Design review of the part built by this model. Coordinates are the model's own, in mm. Face numbers are marked on the shaded views. A direction names the side the tool comes from. Give positions to 0.01 mm unless a question says otherwise; leave off trailing zeros. Order: outer loops, then holes, each group sorted by start corner. A loop starts at its lowest first (then second) coordinate and runs counter-clockwise, first axis right, second up. Notation, with made-up numbers: (64, 38) -> (116, 38) arc R9 ccw to (116, 47) -> close; hole circle Ø11 at (73.5, -27.75). An arc over 180 degrees is marked (long way). Use a Markdown table: item, result. Add a question column.
```python
from build123d import *

# Parameters (mm, degrees)
SKETCH1_W           = 20
SKETCH1_H           = 15
BOSS_EXTRUDE1_DEPTH = 2.54
SKETCH2_W           = 20
SKETCH2_H           = 2.54
BOSS_EXTRUDE2_DEPTH = 10.16
CUT_EXTRUDE1_REACH  = 20.933
SKETCH3_R           = 2.4765
FILLET1_R           = 2.54
SKETCH4_R           = 0.5
CUT_EXTRUDE2_DEPTH  = 10


with BuildPart() as part:
    # Sketch1 → Boss-Extrude1 (new body)
    with BuildSketch(Plane.XY):
        with Locations((0, 7.5)):
            Rectangle(SKETCH1_W, SKETCH1_H)
    extrude(amount=BOSS_EXTRUDE1_DEPTH)

    # Sketch2 → Boss-Extrude2 (add)
    with BuildSketch(Plane(origin=(0, 0, 0), x_dir=(-1, 0, 0), z_dir=(0, 0, -1))):
        with Locations((0, 1.27)):
            Rectangle(SKETCH2_W, SKETCH2_H)
    extrude(amount=BOSS_EXTRUDE2_DEPTH)

    # Sketch3 → Cut-Extrude1 (cut, up to next)
    with BuildSketch(Plane(origin=(0, 2.54, 0), x_dir=(1, 0, 0), z_dir=(0, 1, 0)), mode=Mode.PRIVATE) as cut_extrude1_sk1:
        with Locations(Location((0, 5.08, 0), (0, 0, 180))):
            Circle(SKETCH3_R)
    cut_extrude1_tool1 = extrude(cut_extrude1_sk1.sketch, amount=-CUT_EXTRUDE1_REACH, mode=Mode.PRIVATE) & part.part
    add(cut_extrude1_tool1.solids().sort_by_distance((0, 2.54, -5.08))[0], mode=Mode.SUBTRACT)

    # Fillet1
    fillet1_edges = [part.edges().sort_by_distance(p)[0] for p in [
        (0, 2.54, 0),
    ]]
    fillet(fillet1_edges, radius=FILLET1_R)

    # Sketch4 → Cut-Extrude2 (cut)
    with BuildSketch(Plane(origin=(0, 2.54, 0), x_dir=(1, 0, 0), z_dir=(0, 1, 0))):
        with Locations(Location((-8.35, 5.08, 0), (0, 0, 180))):
            Circle(SKETCH4_R)
        with Locations(Location((-4.35, 5.08, 0), (0, 0, 180))):
            Circle(SKETCH4_R)
        with Locations(Location((4.95, 5.08, 0), (0, 0, 180))):
            Circle(SKETCH4_R)
        with Locations(Location((8.95, 5.08, 0), (0, 0, 180))):
            Circle(SKETCH4_R)
    extrude(amount=-CUT_EXTRUDE2_DEPTH, mode=Mode.SUBTRACT)


solid = part.part
```
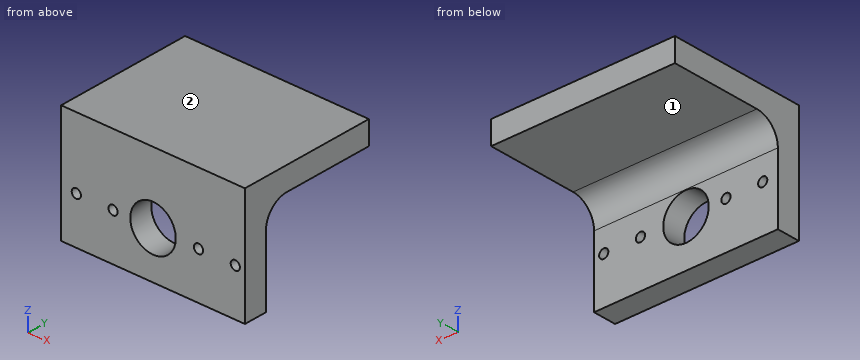
1) For L1, parallel to Z at x = -8.35, y = 1.85; L2, parallel to Z at x = 8.5, y = 12.5, list the stretches that pass through material, from the lowest coordinate up. Write a range as [from, to].
2) Add section C-C (z = -7.25). Give the boundary of the cut face in (x, y), then the cut area to 3 significant figures.
3) Add section D-D (x = 3.25). Give the boundary of the cut face in (y, z).
4) Machinability: for the marked faces 1 and 2, which of the approach directions +Z, -Z, +X, -X, +Y, -Y give a long, thin tool a straight path to every point of the face, cutting with its end or side? Answer none if there is none.
5) Add section B-B (x = -8.35). Give the boundary of the cut face in (y, z).
6) Add section A-A (z = -5.08). Give the boundary of the cut face in (x, y).
7) Insertion check: pin 1 (1 mm diameter, centred on x = 1.5, z = 0, fed in from -Y); pin 2 (1 mm diameter, centred on x = 1.5, y = 6, fed in from -Z). Each pin has a flat end and moves straight along its axis. Give the tip position at first contact, or say it passes through.
Worked answers:
| question | item | result |
|---|---|---|
| 1 | L1 | [-10.16, -5.58], [-4.58, 2.54] |
| 1 | L2 | [0, 2.54] |
| 2 | outline | (-10, 0) -> (-1.19, 0) -> (-1.19, 2.54) -> (-10, 2.54) -> close; (1.19, 0) -> (10, 0) -> (10, 2.54) -> (1.19, 2.54) -> close |
| 2 | area | 44.7 mm^2 |
| 3 | outline | (0, -10.16) -> (2.54, -10.16) -> (2.54, -2.54) arc R2.54 cw to (5.08, 0) -> (15, 0) -> (15, 2.54) -> (0, 2.54) -> close |
| 4 | face 1 | -Z, +X, -X, +Y |
| 4 | face 2 | +Z, +X, -X, +Y, -Y |
| 5 | outline | (0, -10.16) -> (2.54, -10.16) -> (2.54, -5.58) -> (0, -5.58) -> close; (0, -4.58) -> (2.54, -4.58) -> (2.54, -2.54) arc R2.54 cw to (5.08, 0) -> (15, 0) -> (15, 2.54) -> (0, 2.54) -> close |
| 6 | outline | (-10, 0) -> (-8.85, 0) -> (-8.85, 2.54) -> (-10, 2.54) -> close; (-7.85, 0) -> (-4.85, 0) -> (-4.85, 2.54) -> (-7.85, 2.54) -> close; (-3.85, 0) -> (-2.48, 0) -> (-2.48, 2.54) -> (-3.85, 2.54) -> close; (2.48, 0) -> (4.45, 0) -> (4.45, 2.54) -> (2.48, 2.54) -> close; (5.45, 0) -> (8.45, 0) -> (8.45, 2.54) -> (5.45, 2.54) -> close; (9.45, 0) -> (10, 0) -> (10, 2.54) -> (9.45, 2.54) -> close |
| 7 | pin 1 | y = 0 |
| 7 | pin 2 | z = 0 |
